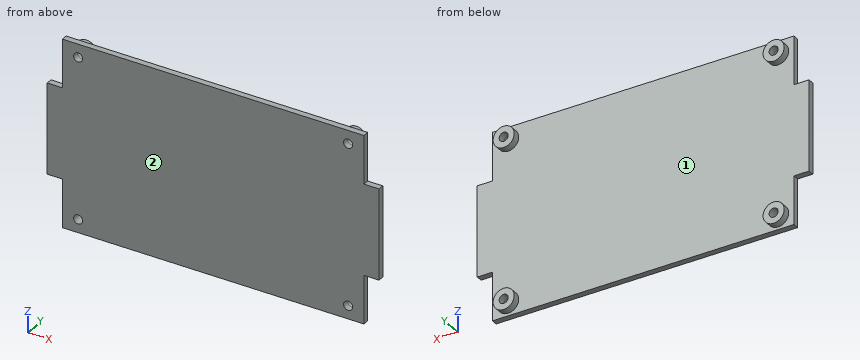
```python
from build123d import *

# Parameters (mm, degrees)
SKETCH_1_W            = 100
SKETCH_1_H            = 62
SKETCH_1_W_2          = 110
SKETCH_1_H_2          = 30
EXTRUDE_466_DEPTH     = 2
SKETCH_2_R            = 1.5
CUT_EXTRUDE_826_DEPTH = 2
SKETCH_3_R            = 3.5
SKETCH_3_R_2          = 1.5
EXTRUDE_1142_DEPTH    = 2.4


with BuildPart() as part:
    # 草图1 → Extrude 466 (new body)
    with BuildSketch(Plane(origin=(0, 0, 0), x_dir=(1, 0, 0), z_dir=(0, 1, 0))):
        Rectangle(SKETCH_1_W, SKETCH_1_H)
        Rectangle(SKETCH_1_W_2, SKETCH_1_H_2)
    extrude(amount=EXTRUDE_466_DEPTH)

    # 草图2 → Cut-Extrude 826 (cut)
    with BuildSketch(Plane(origin=(0, 2, 0), x_dir=(1, 0, 0), z_dir=(0, 1, 0))):
        with Locations((-44.75, 26.65)):
            Circle(SKETCH_2_R)
        with Locations((44.75, 26.65)):
            Circle(SKETCH_2_R)
        with Locations((-44.75, -26.65)):
            Circle(SKETCH_2_R)
        with Locations((44.75, -26.65)):
            Circle(SKETCH_2_R)
    extrude(amount=-CUT_EXTRUDE_826_DEPTH, mode=Mode.SUBTRACT)

    # 草图3 → Extrude 1142 (add)
    with BuildSketch(Plane(origin=(0, 2, 0), x_dir=(1, 0, 0), z_dir=(0, 1, 0))):
        with Locations((-44.75, 26.65)):
            Circle(SKETCH_3_R)
        with Locations((-44.75, 26.65)):
            Circle(SKETCH_3_R_2, mode=Mode.SUBTRACT)
        with Locations((44.75, 26.65)):
            Circle(SKETCH_3_R)
        with Locations((44.75, 26.65)):
            Circle(SKETCH_3_R_2, mode=Mode.SUBTRACT)
        with Locations((-44.75, -26.65)):
            Circle(SKETCH_3_R)
        with Locations((-44.75, -26.65)):
            Circle(SKETCH_3_R_2, mode=Mode.SUBTRACT)
        with Locations((44.75, -26.65)):
            Circle(SKETCH_3_R)
        with Locations((44.75, -26.65)):
            Circle(SKETCH_3_R_2, mode=Mode.SUBTRACT)
    extrude(amount=EXTRUDE_1142_DEPTH)


solid = part.part
```
Geometry: final body of the model. Coordinates: model frame, mm. Face numbers are marked on the shaded views. Coordinates: 2 decimals unless noted, no trailing zeros. Order: outer loops, then holes, each group sorted by start corner. A loop starts at its lowest first (then second) coordinate and runs counter-clockwise, first axis right, second up. Notation, with made-up numbers: (-8.75, 18.5) -> (-4.75, 18.5) arc R5 ccw to (-4.75, 27.5) -> close; hole circle Ø3 at (79, -25.75). An arc over 180 degrees is marked (long way). Write item = value, one per line.
(1) Cut plane D-D on x = -6. Return loops of the section in (y, z), plus the area to 3 significant figures.
Solved:
outline = (0, -31) -> (2, -31) -> (2, 31) -> (0, 31) -> close
area = 124 mm²
(2) Pin query (flat end, axial travel): pin 1 Ø2 at (y, z) = (0.5, -24.5) entering from -X; pin 2 Ø1 at (x, y) = (-51.5, 1) entering from +Z; pin 3 Ø10 at (x, z) = (9, -23) entering from +Y; pin 4 Ø2.5 at (x, z) = (44.75, 26.65) entering from +Y. Return the tip coordinate at first contact, or that it passes through.
Solved:
pin_1 = -50
pin_2 = 15
pin_3 = 2
pin_4 = through
(3) Pull-direction query (X, two-part tool) for the marked faces 1 and 2; classes: pulls with the +X half, pulls with the -X half, needs draft (parallel to the pull), parting line crosses it, or undercut.
Solved:
face_1 = undercut
face_2 = needs draft
(4) Line query: line 1 (X direction, y = 3.25, z = -26.65); line 2 (X direction, y = 1.7, z = -26.65); line 3 (Z direction, x = 44.75, y = 2.6). Output: solid intervals per line, ascending.
Solved:
line_1 = -48.25 to -46.25, -43.25 to -41.25, 41.25 to 43.25, 46.25 to 48.25
line_2 = -50 to -46.25, -43.25 to 43.25, 46.25 to 50
line_3 = -30.15 to -28.15, -25.15 to -23.15, 23.15 to 25.15, 28.15 to 30.15
(5) Cut plane C-C on x = -44.75. Return loops of the section in (y, z), plus the area to 3 significant figures.
Solved:
outline = (0, -31) -> (2, -31) -> (2, -30.15) -> (4.4, -30.15) -> (4.4, -28.15) -> (0, -28.15) -> close; (0, -25.15) -> (4.4, -25.15) -> (4.4, -23.15) -> (2, -23.15) -> (2, 23.15) -> (4.4, 23.15) -> (4.4, 25.15) -> (0, 25.15) -> close; (0, 28.15) -> (4.4, 28.15) -> (4.4, 30.15) -> (2, 30.15) -> (2, 31) -> (0, 31) -> close
area = 131 mm²
(6) Cut plane A-A on y = 3.2. Return loops of the section in (x, z), plus the area to 3 significant figures.
Solved:
outline = circle Ø7 at (-44.75, -26.65); circle Ø7 at (-44.75, 26.65); circle Ø7 at (44.75, -26.65); circle Ø7 at (44.75, 26.65); hole circle Ø3 at (-44.75, -26.65); hole circle Ø3 at (-44.75, 26.65); hole circle Ø3 at (44.75, -26.65); hole circle Ø3 at (44.75, 26.65)
area = 126 mm²
(7) Cut plane B-B on z = -26.65. Return loops of the section in (x, y).
Solved:
outline = (-50, 0) -> (-46.25, 0) -> (-46.25, 4.4) -> (-48.25, 4.4) -> (-48.25, 2) -> (-50, 2) -> close; (-43.25, 0) -> (43.25, 0) -> (43.25, 4.4) -> (41.25, 4.4) -> (41.25, 2) -> (-41.25, 2) -> (-41.25, 4.4) -> (-43.25, 4.4) -> close; (46.25, 0) -> (50, 0) -> (50, 2) -> (48.25, 2) -> (48.25, 4.4) -> (46.25, 4.4) -> close
